```python
from build123d import *

# Parameters (mm, degrees)
SKETCH1_W                      = 50
SKETCH1_H                      = 3
BOSS_EXTRUDE1_DEPTH            = 130
M3_CLEARANCE_HOLE2_D           = 3.4
M3_CLEARANCE_HOLE2_CSINK_D     = 3.45
M3_CLEARANCE_HOLE2_CSINK_ANGLE = 90
SKETCH7_W                      = 21.804410209
SKETCH7_H                      = 3.710121499
BOSS_EXTRUDE2_DEPTH            = 3
CUT_EXTRUDE1_DEPTH             = 141.690312744
M3_CLEARANCE_HOLE3_D           = 3.6


with BuildPart() as part:
    # Sketch1 → Boss-Extrude1 (new body)
    with BuildSketch(Plane(origin=(0, 0, 0), x_dir=(0, 0, -1), z_dir=(1, 0, 0))):
        with Locations((28.71, 1.5)):
            Rectangle(SKETCH1_W, SKETCH1_H)
    extrude(amount=BOSS_EXTRUDE1_DEPTH)

    # M3 Clearance Hole2 (through all)
    with Locations(Plane(origin=(0, 3, 0), x_dir=(1, 0, 0), z_dir=(0, 1, 0))):
        with Locations((80, 18.71), (50, 43.71), (80, 43.71), (50, 18.71)):
            CounterSinkHole(M3_CLEARANCE_HOLE2_D / 2, M3_CLEARANCE_HOLE2_CSINK_D / 2, counter_sink_angle=M3_CLEARANCE_HOLE2_CSINK_ANGLE)

    # Sketch7 → Boss-Extrude2 (add)
    with BuildSketch(Plane.XZ):
        with Locations((119.097794896, -1.854939251)):
            Rectangle(SKETCH7_W, SKETCH7_H)
        with Locations((10.902205105, -1.854939251)):
            Rectangle(SKETCH7_W, SKETCH7_H)
    extrude(amount=-BOSS_EXTRUDE2_DEPTH)

    # Sketch9 → Cut-Extrude1 (cut, through all)
    # profile 1 of 2: a face of its own
    with BuildSketch(Plane(origin=(0, 3, 0), x_dir=(1, 0, 0), z_dir=(0, 1, 0))):
        Polygon((102.295589791, 0.840390735), (102.295589791, 10.639411436), (113.496480192, 10.53967858), (120.695589791, 10.53967858), (120.695589791, -4.617254568), align=None)
        Polygon((120.495589791, 10.33967858), (113.495589791, 10.33967858), (102.495589791, 10.437622706), (102.495589791, 0.989680888), (120.495589791, -4.349319951), align=None, mode=Mode.SUBTRACT)
    # profile 2 of 2: a face of its own
    with BuildSketch(Plane(origin=(0, 3, 0), x_dir=(1, 0, 0), z_dir=(0, 1, 0))):
        Polygon((9.304410209, 10.53967858), (9.304410209, -4.617254568), (27.704410209, 0.840390735), (27.704410209, 10.639411436), (16.503519826, 10.53967858), align=None)
    extrude(amount=-CUT_EXTRUDE1_DEPTH, mode=Mode.SUBTRACT)


with BuildPart() as cut_extrude1_kept_piece:
    # of the separate pieces the step leaves, the one the design keeps (cut_extrude1_pieces_kept)
    add(part.part.solids().sort_by_distance((27.704410209, 3, -3.71))[0])

    # M3 Clearance Hole3 (through all)
    with Locations(Plane(origin=(0, 3, 0), x_dir=(1, 0, 0), z_dir=(0, 1, 0))):
        with Locations((125.269900039, 4.729978462), (125.269900039, 15.269778541), (114.730099961, 15.269778541)):
            m3_clearance_hole3 = Hole(M3_CLEARANCE_HOLE3_D / 2)

    # Mirror1: M3 Clearance Hole3 across plane
    add(m3_clearance_hole3.mirror(Plane(origin=(65, 0, 0), x_dir=(0, 0, 1), z_dir=(1, 0, 0))), mode=Mode.SUBTRACT)


solid = cut_extrude1_kept_piece.part
```
Can you work these out from the model? Positions are in its coordinate system, mm. A direction names the side the tool comes from. Round coordinates to 2 decimals unless told otherwise and drop trailing zeros. Loops run counter-clockwise (first coordinate to the right, second up) from the corner with the lowest first, then second, coordinate; pieces in that order, holes last. Notation, with made-up numbers: M 5,32.5 L 43,32.5 A22 ccw 43,60.5 Z; hole C 66,-9.75 d11. An arc over 180 degrees is marked long. Answer as a JSON object with one key per item and string values. Group by question number.
Q1. Imagine slicing it at C-C, the plane y = 1.2. Count the separate pieces of the cut face and the enclosed holes in it, then the cut area to 3 significant figures.
Q2. Will these pins go through, and if not, where does the flat tip stop? pin 1 (0.9 mm diameter, centred on x = 118.5, y = 2, fed in from +Z); pin 2 (6 mm diameter, centred on x = 125.27, z = -4.73, fed in from -Y); pin 3 (1 mm diameter, centred on x = 65.5, y = 2.5, fed in from +Z).
Q3. We'd pull the mould along Z, two halves only. Please class faces 1 (the cylindrical face through (51.25, 1.47, -44.86)), 2 (the flat face through (125, 1, 0)), 3 (the flat face through (64, 1, -53.71)): +Z half, -Z half, draft (parallel to the pull), parting line (faces both ways), or undercut.
Q4. Imagine slicing it at B-B, the plane z = -18.71. Please give me the cut outline in (x, y) (3 decimals), then the cut area to 3 significant figures.
Q5. On a 3-axis mill with a long thin cutter (end or side, diameter ignored), from which of +Z, -Z, +X, -X, +Y, -Y can I reach the whole of each face in a straight line? I mean faces 4 (the flat face through (117, 2, -10.54)), 5 (the flat face through (64, 0, -26)). Say none if no direction works.
Q6. Please list where these lines run through material, in increasing order: L1, parallel to Z at x = 50, y = 2.2; L2, parallel to X at y = 0.8, z = -15.5; L3, parallel to X at y = 1, z = -43.71.
Q7. Imagine slicing it at A-A, the plane x = 50. Please give me the cut outline in (y, z) (3 decimals), then the cut area to 3 significant figures.
Findings:
{
 "1": {"separate pieces": "1", "enclosed holes": "10", "area": "6,220 mm2"},
 "2": {"pin 1": "stops at z = -10.54", "pin 2": "stops at y = 0", "pin 3": "stops at z = -3.71"},
 "3": {"face 1": "undercut", "face 2": "+Z half", "face 3": "-Z half"},
 "4": {"outline": "M 0,0 L 48.3,0 L 48.3,2.975 L 48.275,3 L 0,3 Z; M 51.7,0 L 78.3,0 L 78.3,2.975 L 78.275,3 L 51.725,3 L 51.7,2.975 Z; M 81.7,0 L 130,0 L 130,3 L 81.725,3 L 81.7,2.975 Z", "area": "370 mm2"},
 "5": {"face 4": "+Z, +Y, -Y", "face 5": "+Z, -Z, +X, -X, -Y"},
 "6": {"L1": "z = -53.71 to -45.41, -42.01 to -20.41, -17.01 to -3.71", "L2": "x = 0 to 2.94, 6.52 to 13.48, 17.06 to 112.94, 116.52 to 123.48, 127.06 to 130", "L3": "x = 0 to 48.3, 51.7 to 78.3, 81.7 to 130"},
 "7": {"outline": "M 0,-53.71 L 3,-53.71 L 3,-45.435 L 2.975,-45.41 L 0,-45.41 Z; M 0,-42.01 L 2.975,-42.01 L 3,-41.985 L 3,-20.435 L 2.975,-20.41 L 0,-20.41 Z; M 0,-17.01 L 2.975,-17.01 L 3,-16.985 L 3,-3.71 L 0,-3.71 Z", "area": "130 mm2"}
}
